```python
from build123d import *

# Parameters (mm, degrees)
SKETCH1_R           = 7.5
BOSS_EXTRUDE1_DEPTH = 10
SKETCH3_R           = 1.55
BOSS_EXTRUDE2_DEPTH = 10
SKETCH4_R           = 6.05
CUT_EXTRUDE2_DEPTH  = 8


with BuildPart() as part:
    # Sketch1 → Boss-Extrude1 (new body)
    with BuildSketch(Plane(origin=(0, 0, 0), x_dir=(1, 0, 0), z_dir=(0, 1, 0))):
        with Locations(Location((0, 0, 0), (0, 0, 270))):
            Circle(SKETCH1_R)
    extrude(amount=BOSS_EXTRUDE1_DEPTH)

    # Sketch3 → Boss-Extrude2 (add)
    # profile 1 of 4: a face of its own
    with BuildSketch(Plane.XZ):
        with BuildLine():
            Line((-5.657484018, 9.350809391), (-3.123198857, 6.818770336))
            ThreePointArc((-3.123198857, 6.818770336), (-5.217761179, 5.387482554), (-6.715339638, 3.339792441))
            Line((-6.715339638, 3.339792441), (-9.191450131, 5.813708387))
            ThreePointArc((-9.191450131, 5.813708387), (-9.193017577, 9.349241945), (-5.657484018, 9.350809391))
        make_face()
        with Locations(Location((-7.424467075, 7.582258889, 0), (0, 0, 270))):
            Circle(SKETCH3_R, mode=Mode.SUBTRACT)
    # profile 2 of 4: a face of its own
    with BuildSketch(Plane.XZ):
        with BuildLine():
            Line((5.813708387, 9.191450131), (3.339792441, 6.715339638))
            ThreePointArc((3.339792441, 6.715339638), (5.387482554, 5.217761179), (6.818770336, 3.123198857))
            Line((6.818770336, 3.123198857), (9.350809391, 5.657484018))
            ThreePointArc((9.350809391, 5.657484018), (9.349241945, 9.193017577), (5.813708387, 9.191450131))
        make_face()
        with Locations(Location((7.582258889, 7.424467075, 0), (0, 0, 270))):
            Circle(SKETCH3_R, mode=Mode.SUBTRACT)
    # profile 3 of 4: a face of its own
    with BuildSketch(Plane.XZ):
        with BuildLine():
            Line((9.191450131, -5.813708387), (6.715339638, -3.339792441))
            ThreePointArc((6.715339638, -3.339792441), (5.217761179, -5.387482554), (3.123198857, -6.818770336))
            Line((3.123198857, -6.818770336), (5.657484018, -9.350809391))
            ThreePointArc((5.657484018, -9.350809391), (9.193017577, -9.349241945), (9.191450131, -5.813708387))
        make_face()
        with Locations(Location((7.424467075, -7.582258889, 0), (0, 0, 270))):
            Circle(SKETCH3_R, mode=Mode.SUBTRACT)
    # profile 4 of 4: a face of its own
    with BuildSketch(Plane.XZ):
        with BuildLine():
            Line((-5.813708387, -9.191450131), (-3.339792441, -6.715339638))
            ThreePointArc((-3.339792441, -6.715339638), (-5.387482554, -5.217761179), (-6.818770336, -3.123198857))
            Line((-6.818770336, -3.123198857), (-9.350809391, -5.657484018))
            ThreePointArc((-9.350809391, -5.657484018), (-9.349241945, -9.193017577), (-5.813708387, -9.191450131))
        make_face()
        with Locations(Location((-7.582258889, -7.424467075, 0), (0, 0, 270))):
            Circle(SKETCH3_R, mode=Mode.SUBTRACT)
    extrude(amount=-BOSS_EXTRUDE2_DEPTH)

    # Sketch4 → Cut-Extrude2 (cut)
    with BuildSketch(Plane.XZ):
        with Locations(Location((0, 0, 0), (0, 0, 270))):
            Circle(SKETCH4_R)
    extrude(amount=-CUT_EXTRUDE2_DEPTH, mode=Mode.SUBTRACT)


solid = part.part
```
The model under review builds one solid part; all positions refer to its coordinate system, in mm. A direction names the side the tool comes from. Round coordinates to 2 decimals unless told otherwise and drop trailing zeros. Write each loop counter-clockwise with the first axis right and the second up, starting at its lowest first coordinate (ties: lowest second). Pieces come first, ordered by that corner, then holes. Notation, with made-up numbers: (84.25, -39.75) - (100.25, -39.75) arc R17 ccw to (100.25, -8.75) - close; hole circle Ø9 at (62, 44). An arc over 180 degrees is marked (long way). Answer as CSV lines item,"result". Start each with the question number.
(1) For faces 1 (the cylindrical face through (1.82, 3.94, -5.77)), 2 (the flat face through (-8.067, 4.93, -4.373)), 3 (the flat face through (4.373, 4.93, -8.067)), list the 3-axis set-ups (+Z, -Z, +X, -X, +Y, -Y) from which the entire face can be reached by the end or side of a thin tool; tool diameter is ignored.
(2) We need section C-C on x = 0. State the section outline as (y, z) points.
(3) For pin 1 Ø12 at (x, z) = (1.5, -2.5) entering from -Y; pin 2 Ø1.9 at (x, z) = (7.42, -7.58) entering from +Y; pin 3 Ø4 at (x, y) = (1, 1) entering from +Z; pin 4 Ø6 at (y, z) = (2, 5) entering from -X, all flat-tipped, find the tip position at first contact; note any pin that passes through.
(4) To check wall thickness, follow line 1 (X direction, y = 4, z = 0); line 2 (X direction, y = 6, z = 8.75); line 3 (Y direction, x = 0, z = 1.5). State the ranges of each line that lie inside material, in increasing order.
(5) We need section B-B on y = 2.5. State the section outline as (x, z) points.
(6) Draft analysis for pull direction X (two halves, no side actions). For faces 4 (the flat face through (0, 8, 0)), 5 (the flat face through (5, 0, -5)), 6 (the flat face through (8.067, 4.93, 4.373)), state which applies: pulls with the +X half, pulls with the -X half, needs draft (parallel to the pull), parting line crosses it, or undercut.
(7) We need section D-D on y = 8.75. State the section outline as (x, z) points, plus the area to 3 significant figures.
(8) We need section A-A on z = -8.5. State the section outline as (x, y) points.
Worked answers:
1,face 1,"-Y"
1,face 2,"-X, +Y, -Y"
1,face 3,"-Z, +Y, -Y"
2,outline,"(0, -7.5) - (10, -7.5) - (10, 7.5) - (0, 7.5) - (0, 6.05) - (8, 6.05) - (8, -6.05) - (0, -6.05) - close"
3,pin 1,"y = 0"
3,pin 2,"through"
3,pin 3,"z = 7.5"
3,pin 4,"x = -9.92"
4,line 1,"-7.5 to -6.05, 6.05 to 7.5"
4,line 2,"-9.63 to -8.44, -6.41 to -5.06, 5.37 to 6.78, 8.39 to 9.7"
4,line 3,"8 to 10"
5,outline,"(-9.35, -5.66) arc R2.5 ccw to (-5.81, -9.19) - (-3.34, -6.72) arc R7.5 ccw to (3.12, -6.82) - (5.66, -9.35) arc R2.5 ccw to (9.19, -5.81) - (6.72, -3.34) arc R7.5 ccw to (6.82, 3.12) - (9.35, 5.66) arc R2.5 ccw to (5.81, 9.19) - (3.34, 6.72) arc R7.5 ccw to (-3.12, 6.82) - (-5.66, 9.35) arc R2.5 ccw to (-9.19, 5.81) - (-6.72, 3.34) arc R7.5 ccw to (-6.82, -3.12) - close; hole circle Ø3.1 at (-7.58, -7.42); hole circle Ø3.1 at (-7.42, 7.58); hole circle Ø12.1 at (0, 0); hole circle Ø3.1 at (7.42, -7.58); hole circle Ø3.1 at (7.58, 7.42)"
6,face 4,"undercut"
6,face 5,"needs draft"
6,face 6,"pulls with the +X half"
7,outline,"(-9.35, -5.66) arc R2.5 ccw to (-5.81, -9.19) - (-3.34, -6.72) arc R7.5 ccw to (3.12, -6.82) - (5.66, -9.35) arc R2.5 ccw to (9.19, -5.81) - (6.72, -3.34) arc R7.5 ccw to (6.82, 3.12) - (9.35, 5.66) arc R2.5 ccw to (5.81, 9.19) - (3.34, 6.72) arc R7.5 ccw to (-3.12, 6.82) - (-5.66, 9.35) arc R2.5 ccw to (-9.19, 5.81) - (-6.72, 3.34) arc R7.5 ccw to (-6.82, -3.12) - close; hole circle Ø3.1 at (-7.58, -7.42); hole circle Ø3.1 at (-7.42, 7.58); hole circle Ø3.1 at (7.42, -7.58); hole circle Ø3.1 at (7.58, 7.42)"
7,area,"251 mm²"
8,outline,"(-9.84, 0) - (-8.7, 0) - (-8.7, 10) - (-9.84, 10) - close; (-6.47, 0) - (-5.12, 0) - (-5.12, 10) - (-6.47, 10) - close; (4.81, 0) - (6.18, 0) - (6.18, 10) - (4.81, 10) - close; (8.67, 0) - (9.75, 0) - (9.75, 10) - (8.67, 10) - close"
